from build123d import *

# Parameters (mm, degrees)
SKETCH_1_W             = 67.5
SKETCH_1_H             = 30.5
SKETCH_1_W_2           = 7.75
SKETCH_1_H_2           = 5
EXTRUDE_1_DEPTH        = 20
SKETCH_1_3_R           = 3.5
CUT_EXTRUDE_1_DEPTH    = 13
SKETCH_1_4_R           = 2.1
CUT_EXTRUDE_2_DEPTH    = 43.090675927
SKETCH_1_5_W           = 10
SKETCH_1_5_H           = 14.25
CUT_EXTRUDE_3_DEPTH    = 6
SKETCH_1_6_W           = 10
SKETCH_1_6_H           = 14.25
CUT_EXTRUDE_4_DEPTH    = 5
SKETCH_2_W             = 6
SKETCH_2_H             = 2
CUT_EXTRUDE_5_DEPTH    = 14.25
SKETCH_3_W             = 46
SKETCH_3_H             = 10
SKETCH_3_R             = 3.5
CUT_EXTRUDE_6_DEPTH    = 7.5
SKETCH_3_3_W           = 46
SKETCH_3_3_H           = 5.1
CUT_EXTRUDE_7_DEPTH    = 9.5
SKETCH_4_W             = 8
SKETCH_4_H             = 10
EXTRUDE_2_DEPTH        = 2.5
HOLE_WIZARD_M4_1_D     = 3.3
HOLE_WIZARD_M4_1_DEPTH = 10.1
HOLE_WIZARD_M4_1_TIP   = 0.991420021


with BuildPart() as part:
    # 草图1 → 凸台-拉伸1 (new body)
    with BuildSketch(Plane(origin=(0, 0, 0), x_dir=(1, 0, 0), z_dir=(0, 1, 0))):
        Rectangle(SKETCH_1_W, SKETCH_1_H)
        with Locations((-28.875, -7.5)):
            Rectangle(SKETCH_1_W_2, SKETCH_1_H_2, mode=Mode.SUBTRACT)
        with Locations((-28.875, 7.5)):
            Rectangle(SKETCH_1_W_2, SKETCH_1_H_2, mode=Mode.SUBTRACT)
        with Locations((28.875, 7.5)):
            Rectangle(SKETCH_1_W_2, SKETCH_1_H_2, mode=Mode.SUBTRACT)
        with Locations((28.875, -7.5)):
            Rectangle(SKETCH_1_W_2, SKETCH_1_H_2, mode=Mode.SUBTRACT)
    extrude(amount=-EXTRUDE_1_DEPTH)

    # 草图1<3> → 切除-拉伸1 (cut)
    with BuildSketch(Plane(origin=(0, 0, 0), x_dir=(1, 0, 0), z_dir=(0, 1, 0))):
        with Locations(Location((-28.25, 0, 0), (0, 0, 270))):
            Circle(SKETCH_1_3_R)
        with Locations(Location((28.25, 0, 0), (0, 0, 270))):
            Circle(SKETCH_1_3_R)
    extrude(amount=-CUT_EXTRUDE_1_DEPTH, mode=Mode.SUBTRACT)

    # 草图1<4> → 切除-拉伸2 (cut, through all)
    with BuildSketch(Plane(origin=(0, 0, 0), x_dir=(1, 0, 0), z_dir=(0, 1, 0))):
        with Locations(Location((-28.25, 0, 0), (0, 0, 270))):
            Circle(SKETCH_1_4_R)
        with Locations(Location((28.25, 0, 0), (0, 0, 90))):
            Circle(SKETCH_1_4_R)
    extrude(amount=-CUT_EXTRUDE_2_DEPTH, mode=Mode.SUBTRACT)

    # 草图1<5> → 切除-拉伸3 (cut)
    with BuildSketch(Plane(origin=(0, 0, 0), x_dir=(1, 0, 0), z_dir=(0, 1, 0))):
        with Locations((-18, -8.125)):
            Rectangle(SKETCH_1_5_W, SKETCH_1_5_H)
        with Locations((-6, -8.125)):
            Rectangle(SKETCH_1_5_W, SKETCH_1_5_H)
        with Locations((6, -8.125)):
            Rectangle(SKETCH_1_5_W, SKETCH_1_5_H)
        with Locations((18, -8.125)):
            Rectangle(SKETCH_1_5_W, SKETCH_1_5_H)
    extrude(amount=-CUT_EXTRUDE_3_DEPTH, mode=Mode.SUBTRACT)

    # 草图1<6> → 切除-拉伸4 (cut)
    with BuildSketch(Plane(origin=(0, 0, 0), x_dir=(1, 0, 0), z_dir=(0, 1, 0))):
        with Locations((-18, 8.125)):
            Rectangle(SKETCH_1_6_W, SKETCH_1_6_H)
        with Locations((-6, 8.125)):
            Rectangle(SKETCH_1_6_W, SKETCH_1_6_H)
        with Locations((6, 8.125)):
            Rectangle(SKETCH_1_6_W, SKETCH_1_6_H)
        with Locations((18, 8.125)):
            Rectangle(SKETCH_1_6_W, SKETCH_1_6_H)
    extrude(amount=-CUT_EXTRUDE_4_DEPTH, mode=Mode.SUBTRACT)

    # 草图2 → 切除-拉伸5 (cut)
    with BuildSketch(Plane.XY.offset(15.25)):
        with Locations((-6, -7)):
            Rectangle(SKETCH_2_W, SKETCH_2_H)
        with Locations((-18, -7)):
            Rectangle(SKETCH_2_W, SKETCH_2_H)
        with Locations((6, -7)):
            Rectangle(SKETCH_2_W, SKETCH_2_H)
        with Locations((18, -7)):
            Rectangle(SKETCH_2_W, SKETCH_2_H)
    extrude(amount=-CUT_EXTRUDE_5_DEPTH, mode=Mode.SUBTRACT)

    # 草图3 → 切除-拉伸6 (cut)
    # profile 1 of 2: a face of its own
    with BuildSketch(Plane.XZ.offset(20)):
        with Locations((0, 8.75)):
            Rectangle(SKETCH_3_W, SKETCH_3_H)
        with Locations(Location((18, 9.25, 0), (0, 0, 270))):
            Circle(SKETCH_3_R, mode=Mode.SUBTRACT)
        with Locations(Location((6, 9.25, 0), (0, 0, 270))):
            Circle(SKETCH_3_R, mode=Mode.SUBTRACT)
        with Locations(Location((-6, 9.25, 0), (0, 0, 270))):
            Circle(SKETCH_3_R, mode=Mode.SUBTRACT)
        with Locations(Location((-18, 9.25, 0), (0, 0, 270))):
            Circle(SKETCH_3_R, mode=Mode.SUBTRACT)
    # profile 2 of 2: a face of its own
    with BuildSketch(Plane.XZ.offset(20)):
        with Locations((0, -8.75)):
            Rectangle(SKETCH_3_W, SKETCH_3_H)
        with Locations(Location((-18, -8.25, 0), (0, 0, 270))):
            Circle(SKETCH_3_R, mode=Mode.SUBTRACT)
        with Locations(Location((18, -8.25, 0), (0, 0, 270))):
            Circle(SKETCH_3_R, mode=Mode.SUBTRACT)
        with Locations(Location((6, -8.25, 0), (0, 0, 270))):
            Circle(SKETCH_3_R, mode=Mode.SUBTRACT)
        with Locations(Location((-6, -8.25, 0), (0, 0, 270))):
            Circle(SKETCH_3_R, mode=Mode.SUBTRACT)
    extrude(amount=-CUT_EXTRUDE_6_DEPTH, mode=Mode.SUBTRACT)

    # 草图3<3> → 切除-拉伸7 (cut)
    with BuildSketch(Plane.XZ.offset(20)):
        Rectangle(SKETCH_3_3_W, SKETCH_3_3_H)
    extrude(amount=-CUT_EXTRUDE_7_DEPTH, mode=Mode.SUBTRACT)

    # 草图4 → 凸台-拉伸2 (add)
    with BuildSketch(Plane.XZ.offset(12.5)):
        with Locations((-18, 8.75)):
            Rectangle(SKETCH_4_W, SKETCH_4_H)
        with Locations((-6, 8.75)):
            Rectangle(SKETCH_4_W, SKETCH_4_H)
        with Locations((6, 8.75)):
            Rectangle(SKETCH_4_W, SKETCH_4_H)
        with Locations((18, 8.75)):
            Rectangle(SKETCH_4_W, SKETCH_4_H)
        with Locations((-6, -8.75)):
            Rectangle(SKETCH_4_W, SKETCH_4_H)
        with Locations((6, -8.75)):
            Rectangle(SKETCH_4_W, SKETCH_4_H)
        with Locations((18, -8.75)):
            Rectangle(SKETCH_4_W, SKETCH_4_H)
        with Locations((-18, -8.75)):
            Rectangle(SKETCH_4_W, SKETCH_4_H)
    extrude(amount=EXTRUDE_2_DEPTH)

    # M4 螺纹孔1
    with Locations(Plane(origin=(0, -5, 0), x_dir=(1, 0, 0), z_dir=(0, 1, 0))):
        with Locations((-18, 9), (-6, 9), (6, 9), (18, 9), (18, -9), (6, -9), (-6, -9), (-18, -9)):
            Hole(HOLE_WIZARD_M4_1_D / 2, depth=HOLE_WIZARD_M4_1_DEPTH)
            with Locations((0, 0, -(HOLE_WIZARD_M4_1_DEPTH + HOLE_WIZARD_M4_1_TIP / 2))):  # 118° drill point
                Cone(0, HOLE_WIZARD_M4_1_D / 2, HOLE_WIZARD_M4_1_TIP, mode=Mode.SUBTRACT)


solid = part.part
The model under review builds one solid part; all positions refer to its coordinate system, in mm. A direction names the side the tool comes from. Coordinates: 2 decimals unless noted, no trailing zeros. Write each loop counter-clockwise with the first axis right and the second up, starting at its lowest first coordinate (ties: lowest second). Pieces come first, ordered by that corner, then holes. Notation, with made-up numbers: (79, 3.5) - (118, 3.5) arc R23 ccw to (118, 37.5) - close; hole circle Ø3 at (68.25, 0). An arc over 180 degrees is marked (long way). Answer as a JSON object with one key per item and string values. Group by question number.
1. To check wall thickness, follow probe 1 along X at (y, z) = (-2.25, 12.5); probe 2 along Z at (x, y) = (18, -11.5); probe 3 along X at (y, z) = (-14.5, 13.5). State the ranges of each line that lie inside material, in increasing order.
2. Add section A-A (x = 28.25). Give the boundary of the cut face in (y, z), plus the area to 3 significant figures.
3. Add section B-B (y = -4.25). Give the number of separate pieces and of enclosed holes in the cut face, plus the area to 3 significant figures.
4. Clearance check with flat-ended pins moving along their axes: pin 1 Ø2.5 at (x, y) = (6, -3) entering from +Z; pin 2 Ø3 at (x, z) = (-3, -8) entering from +Y; pin 3 Ø0.8 at (x, z) = (-22.5, -6.5) entering from -Y. State where each tip first meets the part, or that it passes through.
5. Mouldability with a two-part tool opening along X and no side actions: class faces 1 (the face through (31.72, -6.41, -0.46)), 2 (the face through (0, -20, 3)) as pulls with the +X half, pulls with the -X half, needs draft (parallel to the pull), parting line crosses it, or undercut.
6. Machinability: for faces 3 (the face through (9, -7, 8)), 4 (the face through (29, -10, -10)), 5 (the face through (-11, -2, -8)), 6 (the face through (19.31, -11.6, 10)), 7 (the face through (-15.6, -17.5, 11.8)), which of the approach directions +Z, -Z, +X, -X, +Y, -Y give a long, thin tool a straight path to every point of the face, cutting with its end or side? Answer none if there is none.
Findings:
{
 "1": {"probe 1": "-33.75 to -23, -13 to -11, -1 to 1, 11 to 13, 23 to 33.75", "probe 2": "-15.25 to -10.65, -7.35 to -2.55, 2.55 to 7.35, 10.65 to 15.25", "probe 3": "-33.75 to -23, -22 to -14, -10 to -2, 2 to 10, 14 to 22, 23 to 33.75"},
 "2": {"outline": "(-20, -15.25) - (0, -15.25) - (0, -10) - (-20, -10) - close; (-20, -5) - (0, -5) - (0, -3.5) - (-13, -3.5) - (-13, -2.1) - (-20, -2.1) - close; (-20, 2.1) - (-13, 2.1) - (-13, 3.5) - (0, 3.5) - (0, 5) - (-20, 5) - close; (-20, 10) - (0, 10) - (0, 15.25) - (-20, 15.25) - close", "area": "290 mm²"},
 "3": {"separate pieces": "1", "enclosed holes": "6", "area": "687 mm²"},
 "4": {"pin 1": "z = 1", "pin 2": "y = -5", "pin 3": "y = -12.5"},
 "5": {"face 1": "undercut", "face 2": "needs draft"},
 "6": {"face 3": "+Z, +Y", "face 4": "+Y, -Y", "face 5": "-Z, +Y", "face 6": "+Y", "face 7": "-Y"}
}
